Autodesk Inventor part; units mm, degrees
ref_plane "YZ Plane" through (0, 0, 0) normal (1, 0, 0) x (0, 1, 0)
ref_plane "XZ Plane" through (0, 0, 0) normal (0, 1, 0) x (-1, 0, 0)
ref_plane "XY Plane" through (0, 0, 0) normal (0, 0, 1) x (1, 0, 0)
sketch "スケッチ1" plane through (0, 0, 0) normal (1, 0, 0) x (0, 1, 0)
  circle A0 centre (0, 0) radius 5
  dimension "d0" = 10
extrude "押し出し1" add sketch "スケッチ1" along normal blind 71.5
sketch "スケッチ2" plane through (71.5, 0, 0) normal (1, 0, 0) x (0, 0, -1)
  circle A0 centre (0, 0) radius 3
  line L0 (-2, 5.6235) -> (-2, 0.6448)
  line L1 (-2, 0.6448) -> (2, 0.6448)
  line L2 (2, 0.6448) -> (2, 6.3088)
  line L3 (-2, 5.6235) -> (2, 5.6235)
  point P0 (-2, 2.2361)
  point P1 (2, 2.2361)
  dimension "d3" = 6
  dimension "d4" = 2
  dimension "d5" = 2
extrude "押し出し2" cut sketch "スケッチ2" against normal blind 15
properties part number "RZvector-arm-rotate-v1-Shaft-MM5-Shaft" material "アルミニウム 6061"
For this review, take the finished solid that the model builds, in its own axes (mm). A direction names the side the tool comes from. Coordinates: 2 decimals unless noted, no trailing zeros. Order: outer loops, then holes, each group sorted by start corner. A loop starts at its lowest first (then second) coordinate and runs counter-clockwise, first axis right, second up. Notation, with made-up numbers: (-21.5, 52.25) - (36.5, 52.25) arc R9 cw to (36.5, 61.25) - close; hole circle Ø5 at (-27, -27.5). An arc over 180 degrees is marked (long way). Answer as CSV lines item,"result". Start each with the question number.
1) Add section C-C (x = 11.5). State the section outline as (y, z) points, then the cut area to 3 significant figures.
2) Machinability: for faces 1 (the flat face through (71.5, -2.4, -2.2)), 2 (the flat face through (64, 3, -2)), 3 (the cylindrical face through (64, -3, 0)), which of the approach directions +Z, -Z, +X, -X, +Y, -Y give a long, thin tool a straight path to every point of the face, cutting with its end or side? Answer none if there is none.
3) Add section D-D (z = -3.75). State the section outline as (x, y) points, then the cut area to 3 significant figures.
4) Insertion check: P1, Ø2.5, axis at x = 60.5, y = 4, coming from the +Z side; P2, Ø3, axis at x = 20.5, z = 2, coming from the -Y side; P3, Ø1.5, axis at x = 52.5, z = -1, coming from the +Y side. Each pin has a flat end and moves straight along its axis. Give the tip position at first contact, or say it passes through.
5) Add section A-A (y = 0). State the section outline as (x, z) points.
6) Add section B-B (z = 0). State the section outline as (x, y) points.
7) Draft analysis for pull direction Z (two halves, no side actions). For faces 4 (the flat face through (0, 0, 0)), 5 (the cylindrical face through (35, -5, 0)), 6 (the flat face through (56.5, 1, 0)), state which applies: +Z half, -Z half, draft (parallel to the pull), parting line (faces both ways), or undercut.
8) To check wall thickness, follow line 1 along Z through (x, y) = (67.5, 0); line 2 along Y through (x, z) = (62.5, 0); line 3 along X through (y, z) = (4, -0.25). State the ranges of each line that lie inside material, in increasing order. Write a range as [from, to].
Result:
1,outline,"circle Ø10 at (0, 0)"
1,area,"78.5 mm^2"
2,face 1,"+Z, -Z, +X, +Y, -Y"
2,face 2,"+X, +Y"
2,face 3,"+X"
3,outline,"(0, -3.31) - (71.5, -3.31) - (71.5, 3.31) - (0, 3.31) - close"
3,area,"473 mm^2"
4,P1,"z = 4.18"
4,P2,"y = -4.97"
4,P3,"y = 4.99"
5,outline,"(0, -5) - (71.5, -5) - (71.5, -3) - (56.5, -3) - (56.5, 3) - (71.5, 3) - (71.5, 5) - (0, 5) - close"
6,outline,"(0, -5) - (71.5, -5) - (71.5, -3) - (56.5, -3) - (56.5, 5) - (0, 5) - close"
7,face 4,"draft"
7,face 5,"parting line"
7,face 6,"undercut"
8,line 1,"[-5, -3], [3, 5]"
8,line 2,"[-5, -3]"
8,line 3,"[0, 56.5]"
